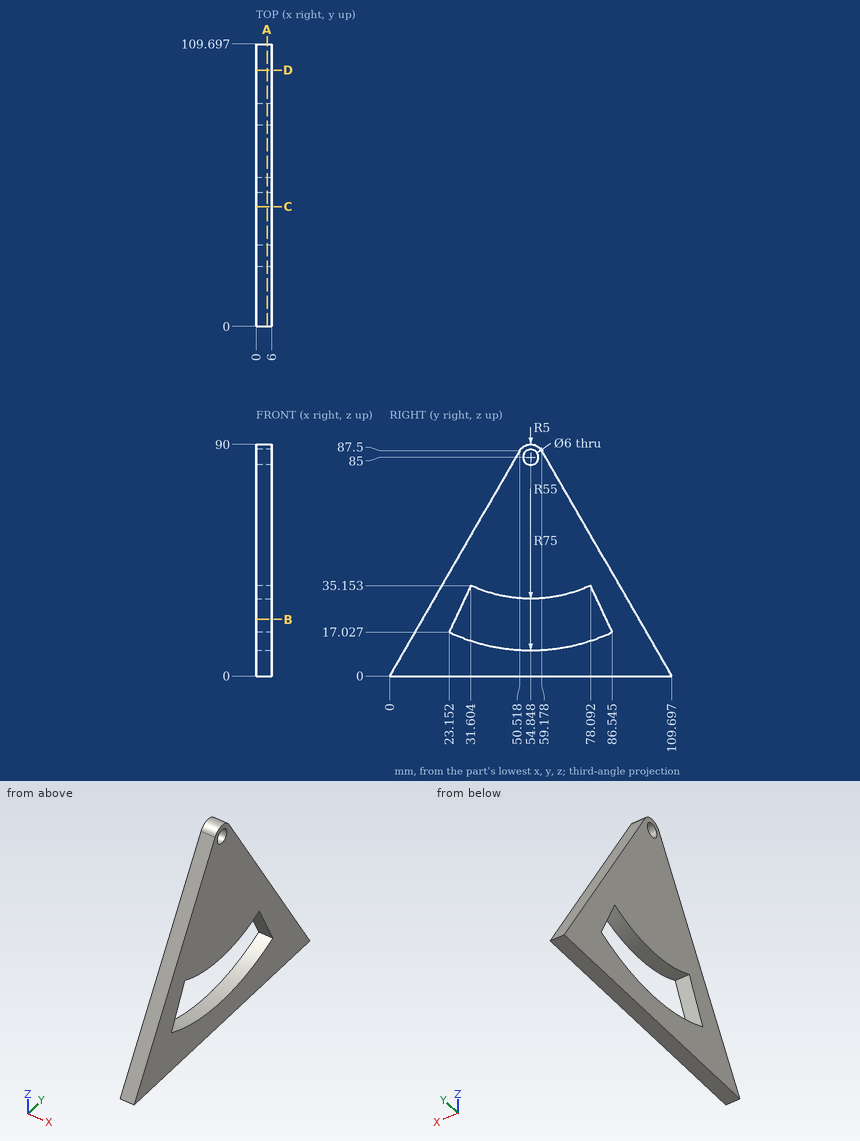
The drawing under review shows one solid part. Ordinate dimensions are in mm from its lowest x, y, z. Round coordinates to 2 decimals unless told otherwise and drop trailing zeros. Write each loop counter-clockwise with the first axis right and the second up, starting at its lowest first coordinate (ties: lowest second). Pieces come first, ordered by that corner, then holes. Notation, with made-up numbers: (37, 69) - (59, 69) arc R20 ccw to (59, 77) - close; hole circle Ø8 at (52, 43). An arc over 180 degrees is marked (long way). Use a Markdown table: item, result. Add a question column.
1. We need section D-D (y = 99.5). State the section outline as (x, z) points, then the cut area to 3 significant figures.
2. We need section A-A (x = 4.25). State the section outline as (y, z) points (1 decimal), then the cut area to 3 significant figures.
3. We need section C-C (y = 46.5). State the section outline as (x, z) points.
4. Wall thickness on probe 1 along Z at (x, y) = (2.1, 55); probe 2 along Z at (x, y) = (2.35, 75.5) (1 decimal); probe 3 along Z at (x, y) = (5.4, 32) (1 decimal): over which ranges is each line inside the solid? List them lowest first.
5. We need section B-B (z = 22). State the section outline as (x, y) points (1 decimal), then the cut area to 3 significant figures.
6. Clearance check with flat-ended pins moving along their axes: pin 1 (1 mm diameter, centred on x = 1.5, y = 27, fed in from +Z); pin 2 (1 mm diameter, centred on x = 3.5, z = 38.5, fed in from +Y); pin 3 (5.5 mm diameter, centred on y = 54.85, z = 85, fed in from -X); pin 4 (1.5 mm diameter, centred on x = 5, z = 75.5, fed in from +Y). State where each tip first meets the part, or that it passes through.
Output:
| question | item | result |
|---|---|---|
| 1 | outline | (0, 0) - (6, 0) - (6, 17.66) - (0, 17.66) - close |
| 1 | area | 106 mm2 |
| 2 | outline | (0, 0) - (109.7, 0) - (59.2, 87.5) arc R5 ccw to (50.5, 87.5) - close; hole (23.2, 17) arc R75 ccw to (86.5, 17) - (78.1, 35.2) arc R55 cw to (31.6, 35.2) - close; hole circle Ø6 at (54.8, 85) |
| 2 | area | 4,030 mm2 |
| 3 | outline | (0, 0) - (6, 0) - (6, 10.47) - (0, 10.47) - close; (0, 30.64) - (6, 30.64) - (6, 80.54) - (0, 80.54) - close |
| 4 | probe 1 | z = 0 to 10, 30 to 82, 88 to 90 |
| 4 | probe 2 | z = 0 to 12.9, 34 to 59.2 |
| 4 | probe 3 | z = 0 to 13.6, 35 to 55.4 |
| 5 | outline | (0, 12.7) - (6, 12.7) - (6, 25.5) - (0, 25.5) - close; (0, 84.2) - (6, 84.2) - (6, 97) - (0, 97) - close |
| 5 | area | 153 mm2 |
| 6 | pin 1 | stops at z = 47.63 |
| 6 | pin 2 | stops at y = 87.76 |
| 6 | pin 3 | passes through |
| 6 | pin 4 | stops at y = 66.54 |
